```python
from build123d import *

# Parameters (mm, degrees)
F1_DEPTH = 5
F2_R     = 2.75
F3_DEPTH = 4.001
F4_R     = 4.99999
F6_DEPTH = 2


# Not quite as in the source:
# - a fillet or chamfer is up to 0.001 mm smaller than in the source, because OpenCascade refuses the exact size


with BuildPart() as f1:
    # F0 (on Right) → F1 (new body, symmetric)
    with BuildSketch(Plane.YZ):
        with BuildLine():
            Line((16.45, 0), (0, 0))
            Line((0, 0), (-5, 0))
            Line((-5, 0), (-5, -4))
            Line((-5, -4), (7.197973195, -4))
            ThreePointArc((7.197973195, -4), (11.4101587327, -1.0428133754), (16.45, 0))
        make_face()
    extrude(amount=F1_DEPTH, both=True)

    # F2 (on face) → F3 (cut, through all)
    with BuildSketch(Plane.XY):
        Circle(F2_R)
    extrude(amount=-F3_DEPTH, mode=Mode.SUBTRACT)

    # F4 (radius 5 in the source; OpenCascade refuses exactly that, so slightly less here)
    f4_edges = [f1.edges().sort_by_distance(p)[0] for p in [
        (5, -5, -2),
        (-5, -5, -2),
    ]]
    fillet(f4_edges, radius=F4_R)

    # F5 (on face) → F6 (join)
    with BuildSketch(Plane.XY):
        with BuildLine():
            Line((-2.75, 16.45), (-2.75, 5.3326822519))
            ThreePointArc((-2.75, 5.3326822519), (0, 6), (2.75, 5.3326822519))
            Line((2.75, 5.3326822519), (2.75, 16.45))
            Line((2.75, 16.45), (-2.75, 16.45))
        make_face()
    extrude(amount=F6_DEPTH)


solid = f1.part
```
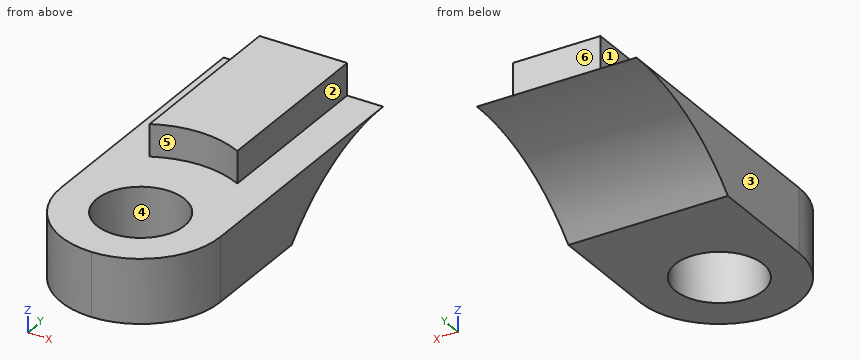
Source: CAD feature listing. Evaluate the final solid. Frame: model axes, mm. Face numbers are marked on the shaded views. A direction names the side the tool comes from. Coordinates: 2 decimals unless noted, no trailing zeros. Loops run counter-clockwise (first coordinate to the right, second up) from the corner with the lowest first, then second, coordinate; pieces in that order, holes last. Notation, with made-up numbers: (-28, 77.5) -> (1, 77.5) arc R24 cw to (1, 107.5) -> close; hole circle Ø10 at (-6, 11.5). An arc over 180 degrees is marked (long way). One line per item, written item: value. Start each with the question number.
Q1. Section query D-D, the plane z = 1.6. Return the cut outline in (x, y), and give its area (3 significant figures).
Q2. Mould query, pull axis Y, two halves, no side actions, for the marked faces 4, 5 and 6. Classes: pulls with the +Y half, pulls with the -Y half, needs draft (parallel to the pull), parting line crosses it, or undercut.
Q3. Section query A-A, the plane x = 0.5. Return the cut outline in (y, z), and give its area (3 significant figures).
Q4. Set-up query: the marked faces 1, 2 and 3. Return all of +Z, -Z, +X, -X, +Y, -Y with unobstructed straight access to the full face (end or side cutting, diameter ignored); none if empty.
Q5. Section query C-C, the plane x = -1. Return the cut outline in (y, z).
Q6. Contact query for flat-ended pins moving along their axis: P1, Ø1.6, axis at y = 9, z = 1, coming from the +X side; P2, Ø1.5, axis at x = 2.5, z = -2, coming from the -Y side. Output: stop coordinate, or through.
Q7. Line query: line 1 along Y through (x, z) = (-1.75, -3.5) (3 decimals); line 2 along Y through (x, z) = (-2, -1.45); line 3 along X through (y, z) = (10, 0.75). Output: solid intervals per line, ascending.
Results:
1. outline: (-2.75, 5.33) arc R6 cw to (2.75, 5.33) -> (2.75, 16.45) -> (-2.75, 16.45) -> close
1. area: 58.7 mm^2
2. face 4: undercut
2. face 5: pulls with the -Y half
2. face 6: pulls with the +Y half
3. outline: (-4.97, -4) -> (-2.7, -4) -> (-2.7, 0) -> (-4.97, 0) -> close; (2.7, -4) -> (7.2, -4) arc R12.7 cw to (16.45, 0) -> (16.45, 2) -> (5.98, 2) -> (5.98, 0) -> (2.7, 0) -> close
3. area: 59.4 mm^2
4. face 1: +Z, -X, +Y, -Y
4. face 2: +Z, +X, +Y, -Y
4. face 3: +Z, -Z, -X, +Y, -Y
5. outline: (-4.9, -4) -> (-2.56, -4) -> (-2.56, 0) -> (-4.9, 0) -> close; (2.56, -4) -> (7.2, -4) arc R12.7 cw to (16.45, 0) -> (16.45, 2) -> (5.92, 2) -> (5.92, 0) -> (2.56, 0) -> close
6. P1: x = 2.75
6. P2: y = -4.68
7. line 1: -4.684 to -2.121, 2.121 to 7.695
7. line 2: -4.58 to -1.89, 1.89 to 10.56
7. line 3: -2.75 to 2.75
